Part model, mm, in its own coordinate system. A direction names the side the tool comes from. Give positions to 0.01 mm unless a question says otherwise; leave off trailing zeros. Write each loop counter-clockwise with the first axis right and the second up, starting at its lowest first coordinate (ties: lowest second). Pieces come first, ordered by that corner, then holes.
```python
from build123d import *

# Parameters (mm, degrees)
BLANKSKE_W           = 27
BLANKSKE_H           = 13.325
BLANK_DEPTH          = 29
TOOTHCUTSIM_DEPTH    = 42.803775248
TEETHCUTS_COUNT      = 8
TEETHCUTS_PITCH      = 3.926990813
CUT_EXTRUDE1_DEPTH   = 6.75
SKETCH3_R            = 5.25
CUT_EXTRUDE2_DEPTH   = 10.25
SKETCH4_R            = 4.5
CUT_EXTRUDE3_DEPTH   = 37.16013862
SKETCH5_R            = 2.5
CUT_EXTRUDE4_DEPTH   = 3.175
SKETCH6_R            = 1.75
CUT_EXTRUDE5_DEPTH   = 40.826953813
MIRROR1_COPY_1_DEPTH = 42.803775248
MIRROR1_COPY_2_DEPTH = 42.803775248
MIRROR1_COPY_3_DEPTH = 42.803775248
MIRROR1_COPY_4_DEPTH = 42.803775248
MIRROR1_COPY_5_DEPTH = 42.803775248
MIRROR1_COPY_6_DEPTH = 42.803775248
MIRROR1_COPY_7_DEPTH = 42.803775248
SKETCH9_W            = 18.526
SKETCH9_H            = 18.526
CUT_EXTRUDE6_DEPTH   = 3.175
SKETCH10_W           = 4.06
SKETCH10_H           = 15.5
BOSS_EXTRUDE2_DEPTH  = 27
SKETCH12_W           = 29
SKETCH12_H           = 6.213309413
SKETCH12_H_2         = 5.066323004
CUT_EXTRUDE7_DEPTH   = 1
SKETCH12_10_R        = 5.25
SKETCH12_10_R_2      = 1.75
CUT_EXTRUDE8_DEPTH   = 7.75
CUT_EXTRUDE9_START   = -7.75
SKETCH12_11_R        = 5.25
SKETCH12_11_R_2      = 1.75
CUT_EXTRUDE9_DEPTH   = 0.75
CHAMFER1_SIZE        = 0.5


with BuildPart() as part:
    # BlankSke → Blank (new body)
    with BuildSketch(Plane.XY):
        with Locations((13.5, 6.6625)):
            Rectangle(BLANKSKE_W, BLANKSKE_H)
    blank = extrude(amount=-BLANK_DEPTH)

    # TooCutSkeSim → ToothCutSim (cut, through all)
    with BuildSketch(Plane.XY):
        Polygon((0.548044212, 10.5125), (-0.548044212, 10.5125), (-1.58095534, 13.3504), (1.58095534, 13.3504), align=None)
    toothcutsim = extrude(amount=-TOOTHCUTSIM_DEPTH, mode=Mode.SUBTRACT)

    # TeethCuts: ToothCutSim ×8
    with Locations(*[(i * TEETHCUTS_PITCH, 0, 0) for i in range(1, TEETHCUTS_COUNT)]):
        add(toothcutsim, mode=Mode.SUBTRACT)

    # Sketch2 → Cut-Extrude1 (cut)
    with BuildSketch(Plane.ZY):
        with BuildLine():
            Line((-7.445049185, 8.763), (-21.554950815, 8.763))
            ThreePointArc((-21.554950815, 8.763), (-24.647184256, 4.857689952), (-25.75, 0))
            Line((-25.75, 0), (-3.25, 0))
            ThreePointArc((-3.25, 0), (-4.352815744, 4.857689952), (-7.445049185, 8.763))
        make_face()
    cut_extrude1 = extrude(amount=-CUT_EXTRUDE1_DEPTH, mode=Mode.SUBTRACT)

    # Sketch3 → Cut-Extrude2 (cut)
    with BuildSketch(Plane.ZY.offset(-6.75)):
        with Locations((-14.5, 0)):
            Circle(SKETCH3_R)
    cut_extrude2 = extrude(amount=-CUT_EXTRUDE2_DEPTH, mode=Mode.SUBTRACT)

    # Sketch4 → Cut-Extrude3 (cut, symmetric)
    with BuildSketch(Plane.ZY.offset(-17)):
        with Locations((-14.5, 0)):
            Circle(SKETCH4_R)
    cut_extrude3 = extrude(amount=CUT_EXTRUDE3_DEPTH, both=True, mode=Mode.SUBTRACT)

    # Sketch5 → Cut-Extrude4 (cut)
    with BuildSketch(Plane(origin=(27, 0, 0), x_dir=(0, 0, -1), z_dir=(1, 0, 0))):
        with Locations((8.932241205, 5.567758795)):
            Circle(SKETCH5_R)
        with Locations((20.067758795, 5.567758795)):
            Circle(SKETCH5_R)
    cut_extrude4 = extrude(amount=-CUT_EXTRUDE4_DEPTH, mode=Mode.SUBTRACT)

    # Sketch6 → Cut-Extrude5 (cut, through all)
    with BuildSketch(Plane(origin=(23.825, 0, 0), x_dir=(0, 0, -1), z_dir=(1, 0, 0))):
        with Locations((20.067758795, 5.567758795)):
            Circle(SKETCH6_R)
        with Locations((8.932241205, 5.567758795)):
            Circle(SKETCH6_R)
    cut_extrude5 = extrude(amount=-CUT_EXTRUDE5_DEPTH, mode=Mode.SUBTRACT)

    # Mirror1: Blank, ToothCutSim, Cut-Extrude1, Cut-Extrude2, Cut-Extrude3, Cut-Extrude4, Cut-Extrude5 across plane
    add(blank.mirror(Plane(origin=(0, 0, -29), x_dir=(0, 0, 1), z_dir=(0, -1, 0))))
    add(toothcutsim.mirror(Plane(origin=(0, 0, -29), x_dir=(0, 0, 1), z_dir=(0, -1, 0))), mode=Mode.SUBTRACT)
    add(cut_extrude1.mirror(Plane(origin=(0, 0, -29), x_dir=(0, 0, 1), z_dir=(0, -1, 0))), mode=Mode.SUBTRACT)
    add(cut_extrude2.mirror(Plane(origin=(0, 0, -29), x_dir=(0, 0, 1), z_dir=(0, -1, 0))), mode=Mode.SUBTRACT)
    add(cut_extrude3.mirror(Plane(origin=(0, 0, -29), x_dir=(0, 0, 1), z_dir=(0, -1, 0))), mode=Mode.SUBTRACT)
    add(cut_extrude4.mirror(Plane(origin=(0, 0, -29), x_dir=(0, 0, 1), z_dir=(0, -1, 0))), mode=Mode.SUBTRACT)
    add(cut_extrude5.mirror(Plane(origin=(0, 0, -29), x_dir=(0, 0, 1), z_dir=(0, -1, 0))), mode=Mode.SUBTRACT)

    # Mirror1 copy 1 sketch → Mirror1 copy 1 (cut, through all)
    with BuildSketch(Plane(origin=(3.926990813, 0, 0), x_dir=(1, 0, 0), z_dir=(0, 0, 1))):
        Polygon((0.548044212, -10.5125), (-0.548044212, -10.5125), (-1.58095534, -13.3504), (1.58095534, -13.3504), align=None)
    extrude(amount=-MIRROR1_COPY_1_DEPTH, mode=Mode.SUBTRACT)

    # Mirror1 copy 2 sketch → Mirror1 copy 2 (cut, through all)
    with BuildSketch(Plane(origin=(7.853981625, 0, 0), x_dir=(1, 0, 0), z_dir=(0, 0, 1))):
        Polygon((0.548044212, -10.5125), (-0.548044212, -10.5125), (-1.58095534, -13.3504), (1.58095534, -13.3504), align=None)
    extrude(amount=-MIRROR1_COPY_2_DEPTH, mode=Mode.SUBTRACT)

    # Mirror1 copy 3 sketch → Mirror1 copy 3 (cut, through all)
    with BuildSketch(Plane(origin=(11.780972438, 0, 0), x_dir=(1, 0, 0), z_dir=(0, 0, 1))):
        Polygon((0.548044212, -10.5125), (-0.548044212, -10.5125), (-1.58095534, -13.3504), (1.58095534, -13.3504), align=None)
    extrude(amount=-MIRROR1_COPY_3_DEPTH, mode=Mode.SUBTRACT)

    # Mirror1 copy 4 sketch → Mirror1 copy 4 (cut, through all)
    with BuildSketch(Plane(origin=(15.70796325, 0, 0), x_dir=(1, 0, 0), z_dir=(0, 0, 1))):
        Polygon((0.548044212, -10.5125), (-0.548044212, -10.5125), (-1.58095534, -13.3504), (1.58095534, -13.3504), align=None)
    extrude(amount=-MIRROR1_COPY_4_DEPTH, mode=Mode.SUBTRACT)

    # Mirror1 copy 5 sketch → Mirror1 copy 5 (cut, through all)
    with BuildSketch(Plane(origin=(19.634954063, 0, 0), x_dir=(1, 0, 0), z_dir=(0, 0, 1))):
        Polygon((0.548044212, -10.5125), (-0.548044212, -10.5125), (-1.58095534, -13.3504), (1.58095534, -13.3504), align=None)
    extrude(amount=-MIRROR1_COPY_5_DEPTH, mode=Mode.SUBTRACT)

    # Mirror1 copy 6 sketch → Mirror1 copy 6 (cut, through all)
    with BuildSketch(Plane(origin=(23.561944875, 0, 0), x_dir=(1, 0, 0), z_dir=(0, 0, 1))):
        Polygon((0.548044212, -10.5125), (-0.548044212, -10.5125), (-1.58095534, -13.3504), (1.58095534, -13.3504), align=None)
    extrude(amount=-MIRROR1_COPY_6_DEPTH, mode=Mode.SUBTRACT)

    # Mirror1 copy 7 sketch → Mirror1 copy 7 (cut, through all)
    with BuildSketch(Plane(origin=(27.488935688, 0, 0), x_dir=(1, 0, 0), z_dir=(0, 0, 1))):
        Polygon((0.548044212, -10.5125), (-0.548044212, -10.5125), (-1.58095534, -13.3504), (1.58095534, -13.3504), align=None)
    extrude(amount=-MIRROR1_COPY_7_DEPTH, mode=Mode.SUBTRACT)

    # Sketch9 → Cut-Extrude6 (cut)
    with BuildSketch(Plane(origin=(27, 0, 0), x_dir=(0, 0, -1), z_dir=(1, 0, 0))):
        with Locations((14.5, 0)):
            Rectangle(SKETCH9_W, SKETCH9_H)
    extrude(amount=-CUT_EXTRUDE6_DEPTH, mode=Mode.SUBTRACT)

    # Sketch10 → Boss-Extrude2 (add, through all)
    with BuildSketch(Plane(origin=(27, 0, 0), x_dir=(0, 0, -1), z_dir=(1, 0, 0))):
        with Locations((31.03, 0)):
            Rectangle(SKETCH10_W, SKETCH10_H)
        with Locations((-2.03, 0)):
            Rectangle(SKETCH10_W, SKETCH10_H)
    extrude(amount=-BOSS_EXTRUDE2_DEPTH)

    # Sketch12 → Cut-Extrude7 (cut)
    with BuildSketch(Plane.ZY):
        with Locations((-14.5, 13.619154707)):
            Rectangle(SKETCH12_W, SKETCH12_H)
        Polygon((0, 10.5125), (-29, 10.5125), (-29, 7.75), (-33.06, 7.75), (-33.06, -7.75), (-29, -7.75), (-29, -10.5125), (0, -10.5125), (0, -7.75), (4.06, -7.75), (4.06, 7.75), (0, 7.75), align=None)
        with BuildLine():
            Line((-21.554950815, 8.763), (-7.445049185, 8.763))
            ThreePointArc((-7.445049185, 8.763), (-3.25, 0), (-7.445049185, -8.763))
            Line((-7.445049185, -8.763), (-21.554950815, -8.763))
            ThreePointArc((-21.554950815, -8.763), (-25.75, 0), (-21.554950815, 8.763))
        make_face(mode=Mode.SUBTRACT)
        with Locations((-14.5, -13.045661502)):
            Rectangle(SKETCH12_W, SKETCH12_H_2)
    extrude(amount=-CUT_EXTRUDE7_DEPTH, mode=Mode.SUBTRACT)

    # Sketch12<10> → Cut-Extrude8 (cut)
    with BuildSketch(Plane.ZY):
        with BuildLine():
            ThreePointArc((-7.445049185, 8.763), (-3.25, 0), (-7.445049185, -8.763))
            Line((-7.445049185, -8.763), (-21.554950815, -8.763))
            ThreePointArc((-21.554950815, -8.763), (-25.75, 0), (-21.554950815, 8.763))
            Line((-21.554950815, 8.763), (-7.445049185, 8.763))
        make_face()
        with Locations((-14.5, 0)):
            Circle(SKETCH12_10_R, mode=Mode.SUBTRACT)
        with Locations(Location((-20.067758795, -5.567758795, 0), (0, 0, 180))):
            Circle(SKETCH12_10_R_2, mode=Mode.SUBTRACT)
        with Locations(Location((-8.932241205, -5.567758795, 0), (0, 0, 180))):
            Circle(SKETCH12_10_R_2, mode=Mode.SUBTRACT)
        with Locations(Location((-8.932241205, 5.567758795, 0), (0, 0, 180))):
            Circle(SKETCH12_10_R_2, mode=Mode.SUBTRACT)
        with Locations(Location((-20.067758795, 5.567758795, 0), (0, 0, 180))):
            Circle(SKETCH12_10_R_2, mode=Mode.SUBTRACT)
    extrude(amount=-CUT_EXTRUDE8_DEPTH, mode=Mode.SUBTRACT)

    # Sketch12<11> → Cut-Extrude9 (cut)
    with BuildSketch(Plane.ZY.offset(CUT_EXTRUDE9_START)):
        with BuildLine():
            ThreePointArc((-7.445049185, 8.763), (-3.25, 0), (-7.445049185, -8.763))
            Line((-7.445049185, -8.763), (-21.554950815, -8.763))
            ThreePointArc((-21.554950815, -8.763), (-25.75, 0), (-21.554950815, 8.763))
            Line((-21.554950815, 8.763), (-7.445049185, 8.763))
        make_face()
        with Locations((-14.5, 0)):
            Circle(SKETCH12_11_R, mode=Mode.SUBTRACT)
        with Locations(Location((-20.067758795, -5.567758795, 0), (0, 0, 180))):
            Circle(SKETCH12_11_R_2, mode=Mode.SUBTRACT)
        with Locations(Location((-8.932241205, -5.567758795, 0), (0, 0, 180))):
            Circle(SKETCH12_11_R_2, mode=Mode.SUBTRACT)
        with Locations(Location((-8.932241205, 5.567758795, 0), (0, 0, 180))):
            Circle(SKETCH12_11_R_2, mode=Mode.SUBTRACT)
        with Locations(Location((-20.067758795, 5.567758795, 0), (0, 0, 180))):
            Circle(SKETCH12_11_R_2, mode=Mode.SUBTRACT)
    extrude(amount=-CUT_EXTRUDE9_DEPTH, mode=Mode.SUBTRACT)

    # Chamfer1
    chamfer1_edges = [part.edges().sort_by_distance(p)[0] for p in [
        (27, 0, -33.06),
        (27, 0, 4.06),
        (14, 7.75, 4.06),
        (14, -7.75, 4.06),
        (14, -7.75, -33.06),
        (14, 7.75, -33.06),
        (1, 0, -33.06),
        (1, 0, 4.06),
    ]]
    chamfer(chamfer1_edges, length=CHAMFER1_SIZE)


solid = part.part
```
1) Wall check: L1, parallel to Z at x = 25.75, y = -2.75; L2, parallel to Y at x = 19.5, z = -14.5; L3, parallel to Y at x = 3.75, z = -6. Give the ranges that are in metal, low to high.
Answers follow:
L1: z = -33.06 to -23.76, -5.24 to 4.06
L2: y = -10.51 to -4.5, 4.5 to 10.51
L3: y = -10.51 to -7.37, 7.37 to 10.51
2) Two-plate mould, pull along Z, no slides. Class faces 4 (the face through (14.655, -11.899, -14.297)), 5 (the face through (14, -10, 0)), 6 (the face through (16.27, 6.09, -21.74)): +Z half, -Z half, draft (parallel to the pull), parting line (faces both ways), or undercut.
Answers follow:
face 4: draft
face 5: +Z half
face 6: undercut
3) Saw through at A-A, the plane y = 0. Write the cut outline in (x, z) (3 decimals).
Answers follow:
outline: (1, -32.56) - (1.5, -33.06) - (26.5, -33.06) - (27, -32.56) - (27, -23.763) - (23.825, -23.763) - (23.825, -19) - (17, -19) - (17, -19.75) - (8.5, -19.75) - (8.5, -25.75) - (1, -25.75) - close; (1, -3.25) - (8.5, -3.25) - (8.5, -9.25) - (17, -9.25) - (17, -10) - (23.825, -10) - (23.825, -5.237) - (27, -5.237) - (27, 3.56) - (26.5, 4.06) - (1.5, 4.06) - (1, 3.56) - close
4) Pin check, flat tips, straight feed: pin 1 Ø4.5 at (y, z) = (-5.57, -8.93) entering from +X (3 decimals); pin 2 Ø4.5 at (x, y) = (10.5, -12) entering from -Z; pin 3 Ø5 at (y, z) = (4, -8) entering from -X. Stop position of each tip, or through.
Answers follow:
pin 1: stops at x = 23.825
pin 2: stops at z = -29
pin 3: stops at x = 8.5
5) 3-axis set-ups, long thin cutter, end or side, ignore diameter. For faces 1 (the face through (8.5, -2, -9)), 2 (the face through (6.8, -11.9, -14.3)), 3 (the face through (12, 10.512, -14)): which of +Z, -Z, +X, -X, +Y, -Y reach the whole face in a straight line?
Answers follow:
face 1: -X
face 2: +Z, -Z, -Y
face 3: +Z, -Z, +Y
6) Saw through at B-B, the plane y = -11. Write the cut outline in (x, z).
Answers follow:
outline: (1, -29) - (3.2, -29) - (3.2, 0) - (1, 0) - close; (4.65, -29) - (7.13, -29) - (7.13, 0) - (4.65, 0) - close; (8.58, -29) - (11.06, -29) - (11.06, 0) - (8.58, 0) - close; (12.51, -29) - (14.98, -29) - (14.98, 0) - (12.51, 0) - close; (16.43, -29) - (18.91, -29) - (18.91, 0) - (16.43, 0) - close; (20.36, -29) - (22.84, -29) - (22.84, 0) - (20.36, 0) - close; (24.29, -29) - (26.76, -29) - (26.76, 0) - (24.29, 0) - close
